Geometry check sheet. Reference: the model listing, model coordinates, mm. A direction names the side the tool comes from. Round coordinates to 2 decimals unless told otherwise and drop trailing zeros. Write each loop counter-clockwise with the first axis right and the second up, starting at its lowest first coordinate (ties: lowest second). Pieces come first, ordered by that corner, then holes. Notation, with made-up numbers: (15.5, 78.25) -> (38.5, 78.25) arc R20 cw to (38.5, 95.25) -> close; hole circle Ø3 at (-37.5, -38.75). An arc over 180 degrees is marked (long way). One line per question, with ' | ' between items.
Autodesk Inventor part; units mm, degrees
ref_plane "Work Plane1" through (1.525, 0, 0) normal (0, 0, 1) x (1, 0, 0)
ref_plane "YZ Plane" through (0, 0, 0) normal (1, 0, 0) x (0, 1, 0)
ref_plane "XZ Plane" through (0, 0, 0) normal (0, 1, 0) x (-1, 0, 0)
sketch "Sketch1" plane through (0, 0, 0) normal (0, 0, 1) x (1, 0, 0)
  line L0 (0, 7.1374) -> (0, 4.9276)
  line L1 (127, 4.7625) -> (152.4, 4.7625)
  line L2 (152.4, 4.7625) -> (152.4, 0)
  line L3 (152.4, 0) -> (-0.0001, 0)
  line L4 (-30.4801, 0) -> (182.88, 0)
  line L5 (-0.0001, 0) -> (-0.0001, 7.1374)
  line L6 (-0.0001, 7.1374) -> (0, 7.1374)
  line L7 (127, 4.7625) -> (123.0311, 4.9276)
  line L8 (123.0311, 4.9276) -> (0, 4.9276)
  line L9 (0, -1.4275) -> (0, 8.5649)
  dimension "d0" = 152.4
  dimension "d1" = 25.4
  dimension "d2" = 9.525
  dimension "d9" = 0.0001
  dimension "d10" = 14.2748
  dimension "d13" = 3.9689
  dimension "d14" = 9.8552
revolve "Body" add sketch "Sketch1" angle 360 about axis through (152.4, 0, 0) along (-1, 0, 0)
sketch "Sketch2" plane through (-0.0001, 0, 0) normal (-1, 0, 0) x (0, 0, 1)
  line L0 (0, 8.2416) -> (7.1374, 4.1208)
  line L1 (7.1374, 4.1208) -> (7.1374, -4.1208)
  line L2 (7.1374, -4.1208) -> (0, -8.2416)
  line L3 (0, -8.2416) -> (-7.1374, -4.1208)
  line L4 (-7.1374, -4.1208) -> (-7.1374, 4.1208)
  line L5 (-7.1374, 4.1208) -> (0, 8.2416)
  point P0 (0, 0)
  point P1 (0, 0)
  dimension "d11" = 14.2748
extrude "Head" add sketch "Sketch2" along normal blind 6.8072
sketch "Sketch4" plane through (0, 0, 0) normal (0, 0, 1) x (1, 0, 0)
  line L0 (-6.8073, 7.1374) -> (-6.8073, 8.2416)
  line L1 (-6.8073, 8.2416) -> (-6.1698, 8.2416)
  line L2 (-6.1698, 8.2416) -> (-6.8073, 7.1374)
  line L3 (-8.1687, 0) -> (1.3613, 0)
  line L4 (-0.0001, 8.2416) -> (-6.8073, 8.2416)
  line L5 (-6.8073, 4.1208) -> (-6.8073, 8.2416)
  dimension "d5" = 30
  dimension "d19" = 14.2748
revolve "Chamfer1" cut sketch "Sketch4" angle 360 about axis through (-10, 0, 0) along (1, 0, 0)
thread "Thread"
chamfer "Chamfer2" distance 0.9739 distance2 0.9447 1 edges at (152.4, -4.7625, 0) measured on face at (152.4, -1.324, 0.065)
ref_plane "Work Plane1" through (1.525, 0, 0) normal (0, 0, 1) x (1, 0, 0)
fillet "Fillet2" radius 0.762 1 edges at (0, -4.9276, 0)
equation "\"d0\" = NLG"
equation "\"d1\" = GEL"
equation "\"d2\" = GD"
equation "\"d10\" = SD2"
equation "\"d14\" = BDM"
equation "\"d11\" = SW"
equation "\"d3\" = KOH - SD"
equation "\"d5\" = ANG1"
equation "\"d19\" = SW0"
equation "\"d63\" = R"
equation "\"d15\" = GEL"
equation "\"d6\" = -0.5 * SPD + 0.5 * GD"
equation "\"NLG\" = 152.4"
equation "\"GD\" = NND"
equation "\"BDM\" = 9.8552"
equation "\"KOH\" = 6.8072"
equation "\"GEL\" = 25.4"
equation "\"SW\" = 14.2748"
equation "\"SW0\" = SW"
equation "\"SPD\" = GD1"
equation "\"SD2\" = SW"
equation "\"SD\" = 0"
equation "\"ANG1\" = 30deg"
equation "\"GAL\" = 3.96875"
equation "\"GUL\" = 0.238 * GAL"
equation "\"R\" = 0.762"
equation "\"d62\" = -NLG - SD + GUL"
equation "\"GD1\" = 7.5773"
equation "\"THREADDIA\" = 9.525"
equation "\"TOA\" = 30deg"
equation "\"NND\" = 9.525"
equation "\"E0\" = 1.155 * SW"
properties part number "ANSI/ASME B18.2.1 - 3/8-16 UNC - 6" material "Steel, Mild"
(1) Material ranges on line 1 (X direction, y = -6.25, z = 2.75); line 2 (Z direction, x = 49.5, y = 2.75); line 3 (Y direction, x = 108, z = -0.25), recorded low to high.
Resolved:
line 1: x = -6.81 to 0 | line 2: z = -4.09 to 4.09 | line 3: y = -4.92 to 4.92
(2) Go/stop test with flat-tipped pins: pin 1 (6 mm diameter, centred on x = 116, z = -1, fed in from +Y); pin 2 (4 mm diameter, centred on x = 16.5, z = -3.5, fed in from -Y); pin 3 (5 mm diameter, centred on x = 109.5, y = -3.5, fed in from +Z). Record where each tip stops, or that it passes through.
Resolved:
pin 1: stops at y = 4.93 | pin 2: stops at y = -4.69 | pin 3: stops at z = 4.83
(3) Access from +Z, -Z, +X, -X, +Y, -Y to the whole of each face (thin tool, end or side, straight path). Record for faces 1 (the cylindrical face through (139.4, -3.78, -2.9)), 2 (the flat face through (-3.36, -6.15, 3.62)).
Resolved:
face 1: +X | face 2: +Z, +X, -X, -Y
(4) Sectioned sample at A-A on x = 82.5. Record the cut outline in (y, z).
Resolved:
outline: circle Ø9.86 at (0, 0)
